```python
from build123d import *

# Parameters (mm, degrees)
F3_D = 50.8


with BuildPart() as f1:
    # F0 (on Top) → F1 (revolve)
    with BuildSketch(Plane.XY):
        Polygon((0, 161.678255), (0, 0), (86.155102, 0), (86.155102, 69.290683), (43.260872, 69.290683), (45.093954, 117.317565), (70.757166, 140.781075), (70.757166, 161.678255), align=None)
    revolve(axis=Axis((0, 80.839127, 0), (0, -1, 0)))

    # F3 (through all)
    with Locations(Plane(origin=(0, 161.678255, 0), x_dir=(-1, 0, 0), z_dir=(0, 1, 0))):
        with Locations((0, 0)):
            Hole(F3_D / 2)


solid = f1.part
```
Verification items for the finished model (mm, model axes). A direction names the side the tool comes from. Give positions to 0.01 mm unless a question says otherwise; leave off trailing zeros. Loops run counter-clockwise (first coordinate to the right, second up) from the corner with the lowest first, then second, coordinate; pieces in that order, holes last. Notation, with made-up numbers: M -18.5,0 L 26.5,0 A34 cw 26.5,31 Z; hole C 20.25,64 d8. An arc over 180 degrees is marked long. Return JSON: item names as keys, results as strings.
1) Mould release check, pull along X, two halves, no side actions. Record for faces 4 (the conical face through (-5.753, 93.64, 43.814)), 5 (the flat face through (30, 161.678, 1)), 6 (the cylindrical face through (-5.506, 79.707, -24.796)): released by +X, released by -X, zero draft, split by the parting line, or undercut.
Findings:
{"face 4": "split by the parting line", "face 5": "zero draft", "face 6": "undercut"}
2) Gauge pin test, flat ends, axial feed: P1, Ø3, axis at x = 24, y = 82.5, coming from the +Z side; P2, Ø1.5, axis at x = -14, y = 126, coming from the -Z side; P3, Ø1, axis at y = 38, z = -58, coming from the +X side. Record the tip position at first contact, or that the pin passes through.
Findings:
{"P1": "stops at z = 37.54", "P2": "stops at z = -53.63", "P3": "stops at x = 64.16"}
3) Section check A-A, the plane y = 40.5. Enter the section's corners in (x, z), and give its area (3 significant figures).
Findings:
{"outline": "C 0,0 d172.31; hole C 0,0 d50.8", "area": "21,300 mm2"}
4) Section check C-C, the plane x = 0. Enter the section's corners in (y, z), and give its area (3 significant figures).
Findings:
{"outline": "M 0,-86.16 L 69.29,-86.16 L 69.29,-43.26 L 117.32,-45.09 L 140.78,-70.76 L 161.68,-70.76 L 161.68,-25.4 L 0,-25.4 Z; M 0,25.4 L 161.68,25.4 L 161.68,70.76 L 140.78,70.76 L 117.32,45.09 L 69.29,43.26 L 69.29,86.16 L 0,86.16 Z", "area": "13,600 mm2"}
5) Tool access check on faces 1 (the flat face through (20, 0, -18)), 2 (the cylindrical face through (-15.339, 151.376, -69.075)), 3 (the flat face through (-20, 69.291, 39)). Record the directions out of +Z, -Z, +X, -X, +Y, -Y that give a thin tool (end or side, any length) a straight path to the whole face; none if there is none.
Findings:
{"face 1": "+Z, -Z, +X, -X, -Y", "face 2": "+Y", "face 3": "none"}
6) Section check B-B, the plane z = 0. Enter the section's corners in (x, y).
Findings:
{"outline": "M -86.16,0 L -25.4,0 L -25.4,161.68 L -70.76,161.68 L -70.76,140.78 L -45.09,117.32 L -43.26,69.29 L -86.16,69.29 Z; M 25.4,0 L 86.16,0 L 86.16,69.29 L 43.26,69.29 L 45.09,117.32 L 70.76,140.78 L 70.76,161.68 L 25.4,161.68 Z"}
7) Material ranges on L1, parallel to Z at x = -0.5, y = 53; L2, parallel to Y at x = 32, z = -76.5; L3, parallel to Y at x = 51, z = -9.5, recorded low to high. Write a range as [from, to].
Findings:
{"L1": "z = [-86.15, -25.4], [25.4, 86.15]", "L2": "y = [0, 69.29]", "L3": "y = [0, 69.29], [123.52, 161.68]"}
